Design review of the part built by this model. Coordinates are the model's own, in mm. A direction names the side the tool comes from. Round coordinates to 2 decimals unless told otherwise and drop trailing zeros. Loops run counter-clockwise (first coordinate to the right, second up) from the corner with the lowest first, then second, coordinate; pieces in that order, holes last. Notation, with made-up numbers: (13.25, 33.5) - (26.25, 33.5) arc R26 cw to (26.25, 55.5) - close; hole circle Ø11 at (-11, 2). An arc over 180 degrees is marked (long way). Return JSON: item names as keys, results as strings. Group by question number.
(1) Clearance check with flat-ended pins moving along their axes: pin 1 (5 mm diameter, centred on x = 14.5, z = -8.5, fed in from -Y); pin 2 (5 mm diameter, centred on y = 21, z = 8.5, fed in from +X); pin 3 (3 mm diameter, centred on x = 60.5, y = 10.5, fed in from +Z). State where each tip first meets the part, or that it passes through.
(2) We need section D-D, the plane y = 8. Write out the cut boundary in (x, z) (3 decimals), and give its area (3 significant figures).
(3) Wall thickness on L1, parallel to X at y = 32.5, z = -8.5; L2, parallel to Y at x = -20, z = 70.5; L3, parallel to X at y = 14, z = -8: over which ranges is each line inside the solid? List them lowest first. Write a range as [from, to].
(4) We need section A-A, the plane x = 0. Write out the cut boundary in (y, z) (3 decimals), and give its area (3 significant figures).
(5) For faces 4 (the flat face through (-8, 15, 24)), 5 (the cylindrical face through (13.08, 30.4, -6.93)), 6 (the cylindrical face through (13.322, 11.352, -11.355)), list the 3-axis set-ups (+Z, -Z, +X, -X, +Y, -Y) from which the entire face can be reached by the end or side of a thin tool; tool diameter is ignored.
(6) The part is to be moulded in two halves that separate along X. For faces 1 (the flat face through (0, 38, 0)), 2 (the flat face through (1.4, 23, 17.9)), 3 (the cylindrical face through (77.336, 4.93, -10.154)), say which applies: pulls with the +X half, pulls with the -X half, needs draft (parallel to the pull), parting line crosses it, or undercut.
(7) We need section C-C, the plane z = 16.51. Write out the cut boundary in (x, y) (3 decimals).
(8) We need section B-B, the plane z = 0. Write out the cut boundary in (x, y), and give its area (3 significant figures).
from build123d import *

# Parameters (mm, degrees)
SKETCH1_R                     = 78
BOSS_EXTRUDE1_DEPTH           = 10
SKETCH2_R                     = 27
BOSS_EXTRUDE2_DEPTH           = 5
SKETCH3_R                     = 25.05
BOSS_EXTRUDE3_DEPTH           = 23
CBORE_FOR_M3_SHCS1_AT_2_COUNT = 2
CBORE_FOR_M3_SHCS1_AT_2_PITCH = 28.596158833
CBORE_FOR_M3_SHCS1_AT_3_COUNT = 2
CBORE_FOR_M3_SHCS1_AT_3_PITCH = 28.596158833


with BuildPart() as part:
    # Sketch1 → Boss-Extrude1 (new body)
    with BuildSketch(Plane(origin=(0, 0, 0), x_dir=(1, 0, 0), z_dir=(0, 1, 0))):
        with Locations(Location((0, 0, 0), (0, 0, 270))):
            Circle(SKETCH1_R)
    extrude(amount=BOSS_EXTRUDE1_DEPTH)

    # Sketch2 → Boss-Extrude2 (add)
    with BuildSketch(Plane(origin=(0, 10, 0), x_dir=(1, 0, 0), z_dir=(0, 1, 0))):
        with Locations(Location((0, 0, 0), (0, 0, 270))):
            Circle(SKETCH2_R)
    extrude(amount=BOSS_EXTRUDE2_DEPTH)

    # Sketch3 → Boss-Extrude3 (add)
    with BuildSketch(Plane(origin=(0, 15, 0), x_dir=(1, 0, 0), z_dir=(0, 1, 0))):
        with Locations(Location((0, 0, 0), (0, 0, 270))):
            Circle(SKETCH3_R)
    extrude(amount=BOSS_EXTRUDE3_DEPTH)

    # Sketch5 → CBORE for M3 SHCS1 (revolve, cut)
    with BuildSketch(Plane(origin=(0, 0, 16.51), x_dir=(0, 0, -1), z_dir=(1, 0, 0))):
        Polygon((0, 0), (0, 38), (1.8, 38), (1.8, 23), (3.25, 23), (3.25, 0.025), (3.275, 0), align=None)
    cbore_for_m3_shcs1 = revolve(axis=Axis((0, -6.35, 16.51), (0, 1, 0)), mode=Mode.SUBTRACT)

    # CBORE for M3 SHCS1 at 2: CBORE for M3 SHCS1 ×2
    with Locations(*[Vector(0.5000000000000012, 0, -0.8660254037844379) * (i * CBORE_FOR_M3_SHCS1_AT_2_PITCH) for i in range(1, CBORE_FOR_M3_SHCS1_AT_2_COUNT)]):
        add(cbore_for_m3_shcs1, mode=Mode.SUBTRACT)

    # CBORE for M3 SHCS1 at 3: CBORE for M3 SHCS1 ×2
    with Locations(*[Vector(-0.4999999999999978, 0, -0.8660254037844399) * (i * CBORE_FOR_M3_SHCS1_AT_3_PITCH) for i in range(1, CBORE_FOR_M3_SHCS1_AT_3_COUNT)]):
        add(cbore_for_m3_shcs1, mode=Mode.SUBTRACT)


solid = part.part
Solutions:
{
 "1": {"pin 1": "y = 23", "pin 2": "x = 24.32", "pin 3": "z = 50.92"},
 "2": {"outline": "circle Ø156 at (0, 0); hole circle Ø6.5 at (-14.298, -8.255); hole circle Ø6.5 at (0, 16.51); hole circle Ø6.5 at (14.298, -8.255)", "area": "19,000 mm^2"},
 "3": {"L1": "[-23.56, -16.08], [-12.51, 12.51], [16.08, 23.56]", "L2": "[0, 10]", "L3": "[-25.79, -17.54], [-11.06, 11.06], [17.54, 25.79]"},
 "4": {"outline": "(0, -78) - (10, -78) - (10, -27) - (15, -27) - (15, -25.05) - (38, -25.05) - (38, 14.71) - (23, 14.71) - (23, 13.26) - (0.025, 13.26) - (0, 13.235) - close; (0, 19.785) - (0.025, 19.76) - (23, 19.76) - (23, 18.31) - (38, 18.31) - (38, 25.05) - (15, 25.05) - (15, 27) - (10, 27) - (10, 78) - (0, 78) - close", "area": "2,780 mm^2"},
 "5": {"face 4": "+Y", "face 5": "+Y, -Y", "face 6": "-Y"},
 "6": {"face 1": "needs draft", "face 2": "undercut", "face 3": "parting line crosses it"},
 "7": {"outline": "(-76.233, 0) - (-3.275, 0) - (-3.25, 0.025) - (-3.25, 23) - (-1.8, 23) - (-1.8, 38) - (-18.839, 38) - (-18.839, 15) - (-21.364, 15) - (-21.364, 10) - (-76.233, 10) - close; (1.8, 23) - (3.25, 23) - (3.25, 0.025) - (3.275, 0) - (76.233, 0) - (76.233, 10) - (21.364, 10) - (21.364, 15) - (18.839, 15) - (18.839, 38) - (1.8, 38) - close"},
 "8": {"outline": "(-78, 0) - (78, 0) - (78, 10) - (27, 10) - (27, 15) - (25.05, 15) - (25.05, 38) - (-25.05, 38) - (-25.05, 15) - (-27, 15) - (-27, 10) - (-78, 10) - close", "area": "2,980 mm^2"}
}
